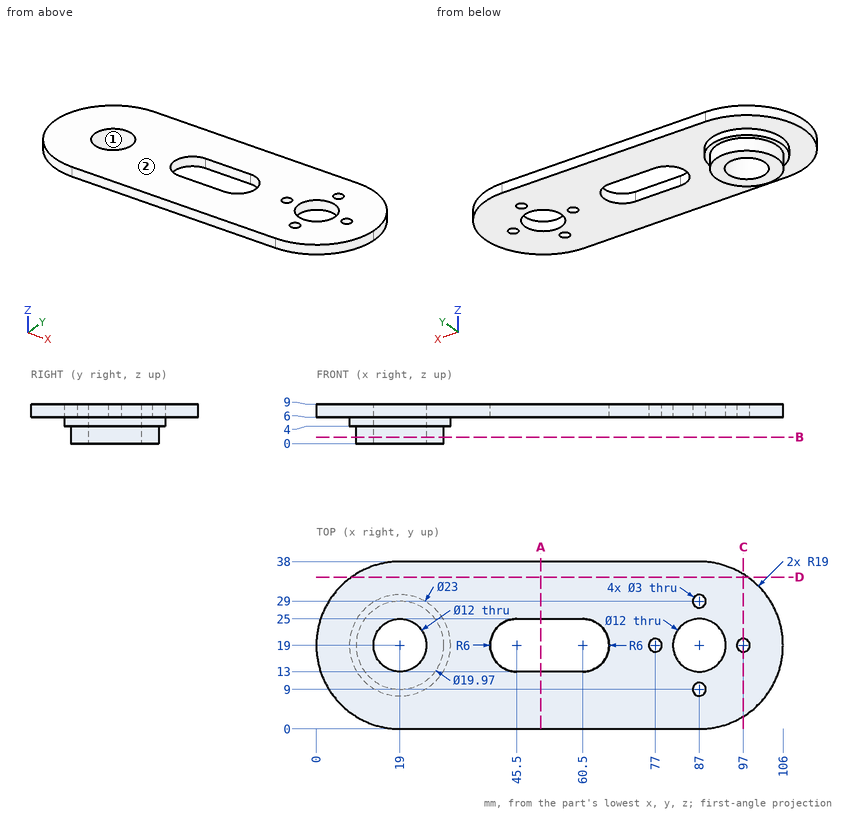
Drawing for the job (mm, zero at the part's lowest x, y, z). Give positions to 0.01 mm unless a question says otherwise; leave off trailing zeros. Order: outer loops, then holes, each group sorted by start corner. A loop starts at its lowest first (then second) coordinate and runs counter-clockwise, first axis right, second up. Notation, with made-up numbers: (-31, 1.5) - (-13, 1.5) arc R14 ccw to (-13, 22.5) - close; hole circle Ø5 at (57, -29). An arc over 180 degrees is marked (long way). Write item = value, one per line. Start each with the question number.
1. Cut at B-B, the plane z = 1.5. List the corners of the cut face in (x, y) (3 decimals).
2. Probe line 1 along Y through (x, z) = (87, 7.6); line 2 along Y through (x, z) = (77, 6.6); line 3 along Z through (x, y) = (26.5, 34). List the from-to ranges inside material, lowest first.
3. Two-plate mould, pull along Y, no slides. Class the marked faces 1 and 2: pulls with the +Y half, pulls with the -Y half, needs draft (parallel to the pull), parting line crosses it, or undercut.
4. Cut at A-A, the plane x = 51. List the corners of the cut face in (y, z), and give its area (3 significant figures).
5. Cut at C-C, the plane x = 97. List the corners of the cut face in (y, z), and give its area (3 significant figures).
6. Cut at D-D, the plane y = 34.5. List the corners of the cut face in (x, z).
7. Drop flat-ended pins along their axis: P1, Ø1.5, axis at y = 7.5, z = 5.5, coming from the +X side; P2, Ø14, axis at x = 87, y = 19, coming from the -Z side; P3, Ø1.5, axis at y = 28.5, z = 7.5, coming from the +X side. Give the stop position or say it passes through.
Taken from the geometry:
q1.outline = circle Ø19.97 at (19, 19); hole circle Ø12 at (19, 19)
q2.line_1 = 0 to 7.5, 10.5 to 13, 25 to 27.5, 30.5 to 38
q2.line_2 = 0 to 17.5, 20.5 to 38
q2.line_3 = 6 to 9
q3.face_1 = undercut
q3.face_2 = needs draft
q4.outline = (0, 6) - (13, 6) - (13, 9) - (0, 9) - close; (25, 6) - (38, 6) - (38, 9) - (25, 9) - close
q4.area = 78.0 mm²
q5.outline = (2.84, 6) - (17.5, 6) - (17.5, 9) - (2.84, 9) - close; (20.5, 6) - (35.16, 6) - (35.16, 9) - (20.5, 9) - close
q5.area = 87.9 mm²
q6.outline = (8.01, 6) - (97.99, 6) - (97.99, 9) - (8.01, 9) - close
q7.P1 = 102.53
q7.P2 = 6
q7.P3 = 103.87
